For this review, take the finished solid that the model builds, in its own axes (mm). A direction names the side the tool comes from. Coordinates: 2 decimals unless noted, no trailing zeros. Order: outer loops, then holes, each group sorted by start corner. A loop starts at its lowest first (then second) coordinate and runs counter-clockwise, first axis right, second up. Notation, with made-up numbers: (-27.75, 31.25) - (28.25, 31.25) arc R18 ccw to (28.25, 57.25) - close; hole circle Ø9 at (-6.75, -3). An arc over 180 degrees is marked (long way). One line per item, written item: value. Start each with the question number.
(1) Clearance check with flat-ended pins moving along their axes: pin 1 (4 mm diameter, centred on y = -20, z = -3, fed in from -X); pin 2 (6.5 mm diameter, centred on y = -16.5, z = -3.5, fed in from +X); pin 3 (5 mm diameter, centred on y = -12.5, z = -25.5, fed in from +X). State where each tip first meets the part, or that it passes through.
(2) Mouldability with a two-part tool opening along Y and no side actions: class faces 1 (the flat face through (-8, -23.283, 0)), 2 (the cylindrical face through (10.222, -10.959, 21.485)), 3 (the flat face through (12, -17, 0)) as released by +Y, released by -Y, zero draft, split by the parting line, or undercut.
(3) Consider section B-B on x = 6. Write out the cut boundary in (y, z).
(4) Consider section D-D on x = 9.5. Write out the cut boundary in (y, z).
(5) Consider section A-A on y = 0. Write out the cut boundary in (x, z).
(6) To check wall thickness, follow line 1 along X through (y, z) = (-13, 12); line 2 along X through (y, z) = (-14.5, -15); line 3 along Y through (x, z) = (9.5, 22). State the ranges of each line that lie inside material, in increasing order.
(7) For faces 4 (the cylindrical face through (-11, 0, 0)), 5 (the flat face through (0, 13.083, 0)), 6 (the flat face through (-12, -17, 0)), list the 3-axis set-ups (+Z, -Z, +X, -X, +Y, -Y) from which the entire face can be reached by the end or side of a thin tool; tool diameter is ignored.
(8) Consider section C-C on z = 0. Write out the cut boundary in (x, y).
```python
from build123d import *

# Parameters (mm, degrees)
BOSS_EXTRUDE1_DEPTH      = 33
BOSS_EXTRUDE1_DEPTH_BACK = 33
SKETCH1_R                = 16
SKETCH1_R_2              = 11
CUT_EXTRUDE1_DEPTH       = 33
BOSS_EXTRUDE2_DEPTH      = 66
CUT_EXTRUDE4_DEPTH       = 72.792049234


with BuildPart() as part:
    # Sketch1 → Boss-Extrude1 (new, two sides: drawn at the far end of the back side and taken through both)
    with BuildSketch(Plane.XY.offset(-BOSS_EXTRUDE1_DEPTH_BACK)):
        Circle(SKETCH1_R)
        Circle(SKETCH1_R_2, mode=Mode.SUBTRACT)
    extrude(amount=BOSS_EXTRUDE1_DEPTH + BOSS_EXTRUDE1_DEPTH_BACK)

    # Sketch2 → Cut-Extrude1 (cut)
    with BuildSketch(Plane.XY.offset(33)):
        Polygon((-3, 10.583005244), (-3, 13.083005244), (0, 13.083005244), (3, 13.083005244), (3, 10.583005244), align=None)
    cut_extrude1 = extrude(amount=-CUT_EXTRUDE1_DEPTH, mode=Mode.SUBTRACT)

    # Mirror2: Cut-Extrude1 across plane
    add(cut_extrude1.mirror(Plane(origin=(0, 0, 0), x_dir=(1, 0, 0), z_dir=(0, 0, -1))), mode=Mode.SUBTRACT)

    # Sketch3 → Boss-Extrude2 (add, through all)
    with BuildSketch(Plane.XY.offset(33)):
        with BuildLine():
            Line((-3, -23.283005244), (-3, -15.716233646))
            ThreePointArc((-3, -15.716233646), (-7.927011319, -13.898290958), (-12, -10.583005244))
            Line((-12, -10.583005244), (-12, -23.283005244))
            Line((-12, -23.283005244), (-3, -23.283005244))
        make_face()
        with BuildLine():
            ThreePointArc((12, -10.583005244), (7.927011319, -13.898290958), (3, -15.716233646))
            Line((3, -15.716233646), (3, -23.283005244))
            Line((3, -23.283005244), (12, -23.283005244))
            Line((12, -23.283005244), (12, -10.583005244))
        make_face()
    extrude(amount=-BOSS_EXTRUDE2_DEPTH)

    # Sketch4 → Cut-Extrude4 (cut, through all)
    with BuildSketch(Plane.XY.offset(33)):
        Polygon((-3, -10.583005244), (-3, -16.271539673), (3, -16.271539673), (3, -15.716233646), (3, -10.583005244), align=None)
    extrude(amount=-CUT_EXTRUDE4_DEPTH, mode=Mode.SUBTRACT)

    # Sketch10 → CBORE for M5 Hex Head Bolt3 (revolve, cut)
    with BuildSketch(Plane(origin=(12, -16.933005244, 20.158167141), x_dir=(0, 0, -1), z_dir=(0, 1, 0))):
        Polygon((0, 0), (0, 11.652366702), (2.75, 10), (2.75, 3.58), (6.12, 3.58), (6.12, 0.025), (6.145, 0), align=None)
    cbore_for_m5_hex_head_bolt3 = revolve(axis=Axis((18.35, -16.933005244, 20.158167141), (-1, 0, 0)), mode=Mode.SUBTRACT)

    # Mirror3: CBORE for M5 Hex Head Bolt3 across plane
    add(cbore_for_m5_hex_head_bolt3.mirror(Plane.XY), mode=Mode.SUBTRACT)

    # Sketch14 → M5x0.8 Tapped Hole1 (revolve, cut)
    with BuildSketch(Plane(origin=(-3, -16.933005244, 20.158167141), x_dir=(0, 0, -1), z_dir=(0, 1, 0))):
        Polygon((0, 0), (0, 13.6618073), (2.1, 12.4), (2.1, 0.425), (2.525, 0), align=None)
    m5x0_8_tapped_hole1 = revolve(axis=Axis((3.35, -16.933005244, 20.158167141), (-1, 0, 0)), mode=Mode.SUBTRACT)

    # Mirror4: M5x0.8 Tapped Hole1 across plane
    add(m5x0_8_tapped_hole1.mirror(Plane.XY), mode=Mode.SUBTRACT)


solid = part.part
```
Geometry check:
1. pin 1: stops at x = -12
1. pin 2: stops at x = 12
1. pin 3: stops at x = 12.49
2. face 1: released by -Y
2. face 2: undercut
2. face 3: zero draft
3. outline: (-23.28, -33) - (-9.22, -33) - (-9.22, 33) - (-23.28, 33) - close; (9.22, -33) - (14.83, -33) - (14.83, 33) - (9.22, 33) - close; hole circle Ø5.5 at (-16.93, -20.16); hole circle Ø5.5 at (-16.93, 20.16)
4. outline: (-23.28, -33) - (-5.55, -33) - (-5.55, 33) - (-23.28, 33) - close; (5.55, -33) - (12.87, -33) - (12.87, 33) - (5.55, 33) - close; hole circle Ø12.24 at (-16.93, -20.16); hole circle Ø12.24 at (-16.93, 20.16)
5. outline: (-16, -33) - (-11, -33) - (-11, 33) - (-16, 33) - close; (11, -33) - (16, -33) - (16, 33) - (11, 33) - close
6. line 1: x = -12 to -3, 3 to 12
6. line 2: x = -12 to -3, 3 to 8.42
6. line 3: y = -23.28 to -22.77, -11.1 to -5.55, 5.55 to 12.87
7. face 4: +Z, -Z
7. face 5: +Z, -Z, -Y
7. face 6: +Z, -Z, -X, -Y
8. outline: (-12, -23.28) - (-3, -23.28) - (-3, -10.58) arc R11 cw to (-3, 10.58) - (-3, 13.08) - (3, 13.08) - (3, 10.58) arc R11 cw to (3, -10.58) - (3, -23.28) - (12, -23.28) - (12, -10.58) arc R16 ccw (long way) to (-12, -10.58) - close
